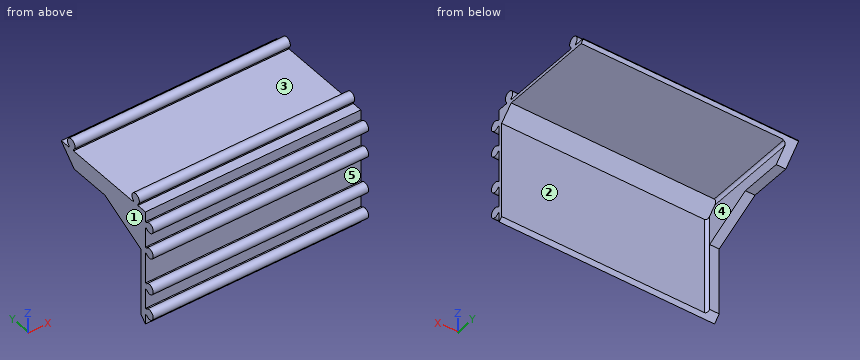
from build123d import *

# Parameters (mm, degrees)
EXTRUDE_1_DEPTH             = 90
SKETCH_2_W                  = 90
SKETCH_2_H                  = 42.75
EXTRUDE_2_DEPTH             = 8.2
SKETCH_3_W                  = 90
SKETCH_3_H                  = 52.45
EXTRUDE_3_DEPTH             = 8.2
SKETCH_4_W                  = 3.95
SKETCH_4_H                  = 2.25
CUT_EXTRUDE_1_DEPTH         = 235.487383722
SKETCH_5_W                  = 3.95
SKETCH_5_H                  = 29.5
CUT_EXTRUDE_2_DEPTH         = 235.487383722
SKETCH_6_W                  = 3.95
SKETCH_6_H                  = 6.2
CUT_EXTRUDE_3_DEPTH         = 235.487383722
SKETCH_7_W                  = 2.25
SKETCH_7_H                  = 3.95
CUT_EXTRUDE_4_DEPTH         = 235.487383722
SKETCH_8_W                  = 4.5
SKETCH_8_H                  = 3.95
CUT_EXTRUDE_5_DEPTH         = 235.487383722
SKETCH_9_W                  = 9
SKETCH_9_H                  = 3.95
CUT_EXTRUDE_6_DEPTH         = 235.487383722
SKETCH_10_W                 = 4.5
SKETCH_10_H                 = 3.95
CUT_EXTRUDE_7_DEPTH         = 235.487383722
SKETCH_11_W                 = 2.25
SKETCH_11_H                 = 3.95
CUT_EXTRUDE_8_DEPTH         = 235.487383722
SKETCH_12_W                 = 45.7
SKETCH_12_H                 = 44.2
CUT_EXTRUDE_9_DEPTH         = 86
HOLE_WIZARD_2_5_2_5_1_D     = 2.5
HOLE_WIZARD_4_5_4_5_1_D     = 4.5
HOLE_WIZARD_8_3_8_3_1_D     = 8.3
HOLE_WIZARD_8_3_8_3_1_DEPTH = 3.2
SKETCH_19_R                 = 1.67252853
SKETCH_19_R_2               = 1.459159852
SKETCH_19_R_3               = 1.459908976
SKETCH_19_R_4               = 1.592821911
SKETCH_19_R_5               = 1.532216665
SKETCH_19_R_6               = 1.596138091
EXTRUDE_4_DEPTH             = 90
CUT_EXTRUDE_START           = -90
SKETCH_20_R                 = 4.15
CUT_EXTRUDE_10_DEPTH        = 90
FILLET_1_R                  = 2
FILLET_2_R                  = 2
FILLET_3_R                  = 2
FILLET_4_R                  = 2
FILLET_5_R                  = 2
FILLET_6_R                  = 2
FILLET_7_R                  = 2
FILLET_8_R                  = 2
FILLET_9_R                  = 2
FILLET_10_R                 = 2
FILLET_11_R                 = 2
FILLET_12_R                 = 2
FILLET_13_R                 = 1.2
CUT_EXTRUDE_11_DEPTH        = 131
EXTRUDE_START               = -4
EXTRUDE_5_DEPTH             = 4
CUT_EXTRUDE_12_DEPTH        = 4
CUT_EXTRUDE_14_DEPTH        = 6
EXTRUDE_6_DEPTH             = 4
EXTRUDE_7_DEPTH             = 87
CUT_EXTRUDE_15_DEPTH        = 84.5


with BuildPart() as part:
    # Эскиз1 → Бобышка-Вытянуть1 (new body)
    with BuildSketch(Plane(origin=(90, 0, 0), x_dir=(0, 0, -1), z_dir=(1, 0, 0))):
        with BuildLine():
            Line((6.75, 160.906238208), (6.75, 204.25))
            Line((6.75, 204.25), (-38.093761792, 204.25))
            ThreePointArc((-38.093761792, 204.25), (-41.825, 203), (-38.093761792, 201.75))
            Line((-38.093761792, 201.75), (-37.5, 201.75))
            Line((-37.5, 201.75), (-37.5, 168.25))
            Line((-37.5, 168.25), (-38.093761792, 168.25))
            ThreePointArc((-38.093761792, 168.25), (-41.825, 167), (-38.093761792, 165.75))
            Line((-38.093761792, 165.75), (-37.5, 165.75))
            Line((-37.5, 165.75), (-37.5, 161.5))
            Line((-37.5, 161.5), (-33.25, 161.5))
            Line((-33.25, 161.5), (-33.25, 160.906238208))
            ThreePointArc((-33.25, 160.906238208), (-32, 157.175), (-30.75, 160.906238208))
            Line((-30.75, 160.906238208), (-30.75, 161.5))
            Line((-30.75, 161.5), (-22.25, 161.5))
            Line((-22.25, 161.5), (-22.25, 160.906238208))
            ThreePointArc((-22.25, 160.906238208), (-21, 157.175), (-19.75, 160.906238208))
            Line((-19.75, 160.906238208), (-19.75, 161.5))
            Line((-19.75, 161.5), (-6.75, 161.5))
            Line((-6.75, 161.5), (-6.75, 160.906238208))
            ThreePointArc((-6.75, 160.906238208), (-5.5, 157.175), (-4.25, 160.906238208))
            Line((-4.25, 160.906238208), (-4.25, 161.5))
            Line((-4.25, 161.5), (4.25, 161.5))
            Line((4.25, 161.5), (4.25, 160.906238208))
            ThreePointArc((4.25, 160.906238208), (5.5, 157.175), (6.75, 160.906238208))
        make_face()
    extrude(amount=-EXTRUDE_1_DEPTH)

    # Эскиз2 → Бобышка-Вытянуть2 (add)
    with BuildSketch(Plane(origin=(0, 0, -6.75), x_dir=(-1, 0, 0), z_dir=(0, 0, -1))):
        with Locations((-45, 182.875)):
            Rectangle(SKETCH_2_W, SKETCH_2_H)
    extrude(amount=EXTRUDE_2_DEPTH)

    # Эскиз3 → Бобышка-Вытянуть3 (add)
    with BuildSketch(Plane(origin=(0, 204.25, 0), x_dir=(-1, 0, 0), z_dir=(0, 1, 0))):
        with Locations((-45, 11.275)):
            Rectangle(SKETCH_3_W, SKETCH_3_H)
    extrude(amount=EXTRUDE_3_DEPTH)

    # Эскиз4 → Вырез-Вытянуть1 (cut, through all)
    with BuildSketch(Plane.ZY):
        with Locations((-12.975, 162.625)):
            Rectangle(SKETCH_4_W, SKETCH_4_H)
    extrude(amount=-CUT_EXTRUDE_1_DEPTH, mode=Mode.SUBTRACT)

    # Эскиз5 → Вырез-Вытянуть2 (cut, through all)
    with BuildSketch(Plane.ZY):
        with Locations((-12.975, 185)):
            Rectangle(SKETCH_5_W, SKETCH_5_H)
    extrude(amount=-CUT_EXTRUDE_2_DEPTH, mode=Mode.SUBTRACT)

    # Эскиз6 → Вырез-Вытянуть3 (cut, through all)
    with BuildSketch(Plane.ZY):
        with Locations((-12.975, 209.35)):
            Rectangle(SKETCH_6_W, SKETCH_6_H)
    extrude(amount=-CUT_EXTRUDE_3_DEPTH, mode=Mode.SUBTRACT)

    # Эскиз7 → Вырез-Вытянуть4 (cut, through all)
    with BuildSketch(Plane.ZY):
        with Locations((-9.875, 210.475)):
            Rectangle(SKETCH_7_W, SKETCH_7_H)
    extrude(amount=-CUT_EXTRUDE_4_DEPTH, mode=Mode.SUBTRACT)

    # Эскиз8 → Вырез-Вытянуть5 (cut, through all)
    with BuildSketch(Plane.ZY):
        with Locations((0, 210.475)):
            Rectangle(SKETCH_8_W, SKETCH_8_H)
    extrude(amount=-CUT_EXTRUDE_5_DEPTH, mode=Mode.SUBTRACT)

    # Эскиз9 → Вырез-Вытянуть6 (cut, through all)
    with BuildSketch(Plane.ZY):
        with Locations((13.25, 210.475)):
            Rectangle(SKETCH_9_W, SKETCH_9_H)
    extrude(amount=-CUT_EXTRUDE_6_DEPTH, mode=Mode.SUBTRACT)

    # Эскиз10 → Вырез-Вытянуть7 (cut, through all)
    with BuildSketch(Plane.ZY):
        with Locations((26.5, 210.475)):
            Rectangle(SKETCH_10_W, SKETCH_10_H)
    extrude(amount=-CUT_EXTRUDE_7_DEPTH, mode=Mode.SUBTRACT)

    # Эскиз11 → Вырез-Вытянуть8 (cut, through all)
    with BuildSketch(Plane.ZY):
        with Locations((36.375, 210.475)):
            Rectangle(SKETCH_11_W, SKETCH_11_H)
    extrude(amount=-CUT_EXTRUDE_8_DEPTH, mode=Mode.SUBTRACT)

    # Эскиз12 → Вырез-Вытянуть9 (cut)
    with BuildSketch(Plane(origin=(90, 0, 0), x_dir=(0, 0, -1), z_dir=(1, 0, 0))):
        with Locations((-13.25, 185)):
            Rectangle(SKETCH_12_W, SKETCH_12_H)
    extrude(amount=-CUT_EXTRUDE_9_DEPTH, mode=Mode.SUBTRACT)

    # Диаметр отверстия Ø2.5 (2.5)1 (through all)
    with Locations(Plane(origin=(90, 0, 0), x_dir=(0, 0, -1), z_dir=(1, 0, 0))):
        with Locations((5.5, 159.25), (-21, 159.25), (-5.5, 159.25), (-32, 159.25), (-39.75, 167), (-39.75, 203)):
            Hole(HOLE_WIZARD_2_5_2_5_1_D / 2)

    # Диаметр отверстия Ø4.5 (4.5)1 (through all)
    with Locations(Plane.ZY):
        with Locations((-13.25, 167), (-13.25, 203), (-5.5, 210.75), (5.5, 210.75), (21, 210.75), (32, 210.75)):
            Hole(HOLE_WIZARD_4_5_4_5_1_D / 2)

    # Диаметр отверстия Ø8.3 (8.3)1
    with Locations(Plane.ZY):
        with Locations((13.25, 185)):
            Hole(HOLE_WIZARD_8_3_8_3_1_D / 2, depth=HOLE_WIZARD_8_3_8_3_1_DEPTH)

    # Эскиз19 → Бобышка-Вытянуть4 (add)
    with BuildSketch(Plane(origin=(90, 0, 0), x_dir=(0, 0, -1), z_dir=(1, 0, 0))):
        with Locations((-39.75, 203)):
            Circle(SKETCH_19_R)
        with Locations((-39.75, 167)):
            Circle(SKETCH_19_R_2)
        with Locations((-32, 159.25)):
            Circle(SKETCH_19_R_3)
        with Locations((-21, 159.25)):
            Circle(SKETCH_19_R_4)
        with Locations((-5.5, 159.25)):
            Circle(SKETCH_19_R_5)
        with Locations((5.5, 159.25)):
            Circle(SKETCH_19_R_6)
    extrude(amount=-EXTRUDE_4_DEPTH)

    # Эскиз20 → Вырез-Вытянуть10 (cut)
    with BuildSketch(Plane.ZY.offset(CUT_EXTRUDE_START)):
        with Locations((13.25, 185)):
            Circle(SKETCH_20_R)
    extrude(amount=CUT_EXTRUDE_10_DEPTH, mode=Mode.SUBTRACT)

    # Скругление1
    fillet_1_edges = [part.edges().sort_by_distance(p)[0] for p in [
        (45, 208.5, -8.75),
    ]]
    fillet(fillet_1_edges, radius=FILLET_1_R)

    # Скругление2
    fillet_2_edges = [part.edges().sort_by_distance(p)[0] for p in [
        (45, 163.75, -11),
    ]]
    fillet(fillet_2_edges, radius=FILLET_2_R)

    # Скругление3
    fillet_3_edges = [part.edges().sort_by_distance(p)[0] for p in [
        (45, 170.25, -11),
    ]]
    fillet(fillet_3_edges, radius=FILLET_3_R)

    # Скругление4
    fillet_4_edges = [part.edges().sort_by_distance(p)[0] for p in [
        (45, 199.75, -11),
    ]]
    fillet(fillet_4_edges, radius=FILLET_4_R)

    # Скругление5
    fillet_5_edges = [part.edges().sort_by_distance(p)[0] for p in [
        (45, 206.25, -11),
    ]]
    fillet(fillet_5_edges, radius=FILLET_5_R)

    # Скругление6
    fillet_6_edges = [part.edges().sort_by_distance(p)[0] for p in [
        (45, 208.5, -2.25),
    ]]
    fillet(fillet_6_edges, radius=FILLET_6_R)

    # Скругление7
    fillet_7_edges = [part.edges().sort_by_distance(p)[0] for p in [
        (45, 208.5, 2.25),
    ]]
    fillet(fillet_7_edges, radius=FILLET_7_R)

    # Скругление8
    fillet_8_edges = [part.edges().sort_by_distance(p)[0] for p in [
        (45, 208.5, 8.75),
    ]]
    fillet(fillet_8_edges, radius=FILLET_8_R)

    # Скругление9
    fillet_9_edges = [part.edges().sort_by_distance(p)[0] for p in [
        (45, 208.5, 17.75),
    ]]
    fillet(fillet_9_edges, radius=FILLET_9_R)

    # Скругление10
    fillet_10_edges = [part.edges().sort_by_distance(p)[0] for p in [
        (45, 208.5, 24.25),
    ]]
    fillet(fillet_10_edges, radius=FILLET_10_R)

    # Скругление11
    fillet_11_edges = [part.edges().sort_by_distance(p)[0] for p in [
        (45, 208.5, 28.75),
    ]]
    fillet(fillet_11_edges, radius=FILLET_11_R)

    # Скругление12
    fillet_12_edges = [part.edges().sort_by_distance(p)[0] for p in [
        (45, 208.5, 35.25),
    ]]
    fillet(fillet_12_edges, radius=FILLET_12_R)

    # Скругление13
    fillet_13_edges = [part.edges().sort_by_distance(p)[0] for p in [
        (4, 185, -9.6),
        (4, 162.9, 13.25),
        (4, 185, 36.1),
        (4, 207.1, 13.25),
    ]]
    fillet(fillet_13_edges, radius=FILLET_13_R)

    # Эскиз21 → Вырез-Вытянуть11 (cut)
    with BuildSketch(Plane(origin=(90, 0, 0), x_dir=(0, 0, -1), z_dir=(1, 0, 0))):
        Polygon((-37.25, 208.5), (11, 161.5), (17.903435656, 161.5), (17.903435656, 214.883320623), (-37.25, 214.883320623), align=None)
    extrude(amount=-CUT_EXTRUDE_11_DEPTH, mode=Mode.SUBTRACT)

    # Эскиз22 → Бобышка-Вытянуть5 (add)
    with BuildSketch(Plane.ZY.offset(EXTRUDE_START)):
        with BuildLine():
            Line((16.161231082, 187.957572246), (10.217049193, 182.167384706))
            ThreePointArc((10.217049193, 182.167384706), (16.145733389, 182.027252425), (16.161231082, 187.957572246))
        make_face()
    extrude(amount=EXTRUDE_5_DEPTH)

    # Эскиз23 → Вырез-Вытянуть12 (cut)
    with BuildSketch(Plane(origin=(4, 0, 0), x_dir=(0, 0, -1), z_dir=(1, 0, 0))):
        Polygon((-29.9, 205.9), (8.330851064, 169.1), (-29.9, 169.1), align=None)
    extrude(amount=-CUT_EXTRUDE_12_DEPTH, mode=Mode.SUBTRACT)

    # Эскиз25 → Вырез-Вытянуть14 (cut)
    with BuildSketch(Plane(origin=(4, 0, 0), x_dir=(0, 0, -1), z_dir=(1, 0, 0))):
        Polygon((-29.9, 164.1), (8.330851064, 164.1), (3.19787234, 169.1), (-29.9, 169.1), align=None)
    extrude(amount=-CUT_EXTRUDE_14_DEPTH, mode=Mode.SUBTRACT)

    # Эскиз26 → Бобышка-Вытянуть6 (add)
    with BuildSketch(Plane(origin=(4, 0, 0), x_dir=(0, 0, -1), z_dir=(1, 0, 0))):
        Polygon((-29.9, 184.1), (-19.75, 164.1), (-29.9, 164.1), align=None)
    extrude(amount=-EXTRUDE_6_DEPTH)

    # Эскиз27 → Бобышка-Вытянуть7 (add)
    with BuildSketch(Plane(origin=(90, 0, 0), x_dir=(0, 0, -1), z_dir=(1, 0, 0))):
        Polygon((-30.75, 162.9), (-36.1, 162.9), (-36.1, 168.25), align=None)
    extrude(amount=-EXTRUDE_7_DEPTH)

    # Эскиз28 → Вырез-Вытянуть15 (cut)
    with BuildSketch(Plane(origin=(90, 0, 0), x_dir=(0, 0, -1), z_dir=(1, 0, 0))):
        Polygon((-36.1, 207.1), (-35.812765957, 207.1), (-36.1, 207.379792746), align=None)
    extrude(amount=-CUT_EXTRUDE_15_DEPTH, mode=Mode.SUBTRACT)


solid = part.part
Here's how the part is built. I have some questions about the finished solid (model axes, mm). Face numbers are marked on the shaded views. A direction names the side the tool comes from. Round coordinates to 2 decimals unless told otherwise and drop trailing zeros. Write each loop counter-clockwise with the first axis right and the second up, starting at its lowest first coordinate (ties: lowest second). Pieces come first, ordered by that corner, then holes. Notation, with made-up numbers: (85, 11) -> (124, 11) arc R16 cw to (124, 41) -> close; hole circle Ø11 at (79, -37.75). An arc over 180 degrees is marked (long way). One line per item, written item: value.
1) We'd pull the mould along Y, two halves only. Please class the marked faces 1, 2 and 3: released by +Y, released by -Y, zero draft, split by the parting line, or undercut.
Filled sheet:
face 1: zero draft
face 2: released by +Y
face 3: undercut
2) I'm going to push flat-ended pins straight in: pin 1 Ø0.5 at (x, y) = (42.5, 161) entering from +Z; pin 2 Ø2 at (x, y) = (11.5, 175.5) entering from +Z; pin 3 Ø2 at (y, z) = (175.5, 24) entering from -X; pin 4 Ø2 at (x, y) = (41, 205.5) entering from +Z. Where does each tip first touch, or does it pass through?
Filled sheet:
pin 1: stops at z = 33.43
pin 2: stops at z = 37.5
pin 3: passes through
pin 4: stops at z = 41.18
3) For the marked faces 4 and 5, which set-ups out of +Z, -Z, +X, -X, +Y, -Y let a thin tool reach every point of the face, with its end or its side?
Filled sheet:
face 4: -Z, +X, +Y
face 5: +X, -X
4) Suppose I cut it at D-D on y = 187.5. List the corners of the cut face in (x, z) for me.
Filled sheet:
outline: (0, 29.9) -> (4, 29.9) -> (4, 34.9) arc R1.2 cw to (5.2, 36.1) -> (90, 36.1) -> (90, 37.5) -> (0, 37.5) -> close
5) Suppose I cut it at A-A on z = 39.75. List the corners of the cut face in (x, y) for me (3 decimals), plus the area to 3 significant figures.
Filled sheet:
outline: (0, 164.925) -> (90, 164.925) -> (90, 169.075) -> (0, 169.075) -> close; (0, 200.925) -> (90, 200.925) -> (90, 205.075) -> (0, 205.075) -> close
area: 747 mm2
6) If I drill on line 1 (Z direction, x = 71, y = 161); line 2 (Y direction, x = 50, z = 13.5); line 3 (Z direction, x = 24, y = 183), over which ranges is the centre line in solid material (lowest first)? Write a range as [from, to].
Filled sheet:
line 1: z = [-6.75, -4.25], [4.25, 6.75], [19.75, 22.25], [30.75, 33.25]
line 2: y = [161.5, 162.9]
line 3: z = [36.1, 37.5]
7) Suppose I cut it at B-B on y = 159.25. List the corners of the cut face in (x, z) for me (3 decimals).
Filled sheet:
outline: (0, -7.575) -> (90, -7.575) -> (90, -3.425) -> (0, -3.425) -> close; (0, 3.425) -> (90, 3.425) -> (90, 7.575) -> (0, 7.575) -> close; (0, 18.925) -> (90, 18.925) -> (90, 23.075) -> (0, 23.075) -> close; (0, 29.925) -> (90, 29.925) -> (90, 34.075) -> (0, 34.075) -> close
